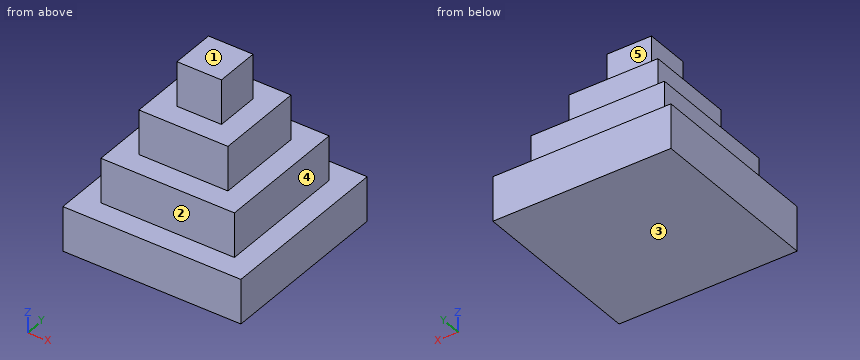
```python
from build123d import *

# Parameters (mm, degrees)
F1_W     = 25
F1_H     = 25
F1_W_2   = 18.75
F1_H_2   = 18.75
F2_DEPTH = 6.25
F1_W_3   = 12.5
F1_H_3   = 12.5
F3_DEPTH = 12.5
F1_W_4   = 6.25
F1_H_4   = 6.25
F4_DEPTH = 18.75
F5_DEPTH = 25


with BuildPart() as f2:
    # F1 (on Top) → F2 (new body)
    with BuildSketch(Plane.XY):
        with Locations((12.5, 12.5)):
            Rectangle(F1_W, F1_H)
        with Locations((12.5, 12.5)):
            Rectangle(F1_W_2, F1_H_2, mode=Mode.SUBTRACT)
    extrude(amount=F2_DEPTH)

    # F1 (on Top) → F3 (join)
    with BuildSketch(Plane.XY):
        with Locations((12.5, 12.5)):
            Rectangle(F1_W_2, F1_H_2)
        with Locations((12.5, 12.5)):
            Rectangle(F1_W_3, F1_H_3, mode=Mode.SUBTRACT)
    extrude(amount=F3_DEPTH)

    # F1 (on Top) → F4 (join)
    with BuildSketch(Plane.XY):
        with Locations((12.5, 12.5)):
            Rectangle(F1_W_3, F1_H_3)
        with Locations((12.5, 12.5)):
            Rectangle(F1_W_4, F1_H_4, mode=Mode.SUBTRACT)
    extrude(amount=F4_DEPTH)

    # F1 (on Top) → F5 (join)
    with BuildSketch(Plane.XY):
        with Locations((12.5, 12.5)):
            Rectangle(F1_W_4, F1_H_4)
    extrude(amount=F5_DEPTH)


solid = f2.part
```
Work out the finished part from the listing and answer in its coordinate system (mm). Face numbers are marked on the shaded views. A direction names the side the tool comes from. Round coordinates to 2 decimals unless told otherwise and drop trailing zeros. Order: outer loops, then holes, each group sorted by start corner. A loop starts at its lowest first (then second) coordinate and runs counter-clockwise, first axis right, second up.
Q1. Given pin 1 Ø3 at (x, y) = (4, 8.5) entering from +Z; pin 2 Ø1 at (x, z) = (14.5, 20) entering from +Y (3 decimals); pin 3 Ø5 at (y, z) = (12.5, 23.5) entering from +X (3 decimals), each flat-ended and moving along its own axis, determine where each tip first touches the part or whether it passes through.
Solution:
pin 1: stops at z = 12.5
pin 2: stops at y = 15.625
pin 3: stops at x = 15.625
Q2. Find the intervals of material crossed by line 1 along Z through (x, y) = (4, 22); line 2 along X through (y, z) = (10.5, 6.75) (3 decimals), in increasing order.
Solution:
line 1: z = 0 to 6.25
line 2: x = 3.125 to 21.875
Q3. A cutting plane is placed at A-A, the plane y = 18.25. Determine the outline of the cut face in (x, z) (3 decimals), then the cut area to 3 significant figures.
Solution:
outline: (0, 0) - (25, 0) - (25, 6.25) - (21.875, 6.25) - (21.875, 12.5) - (18.75, 12.5) - (18.75, 18.75) - (6.25, 18.75) - (6.25, 12.5) - (3.125, 12.5) - (3.125, 6.25) - (0, 6.25) - close
area: 352 mm2
Q4. A cutting plane is placed at B-B, the plane x = 12.5. Determine the outline of the cut face in (y, z) (3 decimals).
Solution:
outline: (0, 0) - (25, 0) - (25, 6.25) - (21.875, 6.25) - (21.875, 12.5) - (18.75, 12.5) - (18.75, 18.75) - (15.625, 18.75) - (15.625, 25) - (9.375, 25) - (9.375, 18.75) - (6.25, 18.75) - (6.25, 12.5) - (3.125, 12.5) - (3.125, 6.25) - (0, 6.25) - close
Q5. A tool of negligible diameter and unlimited length cuts with its end or side. For the marked faces 1, 2, 3, 4 and 5, from which of +Z, -Z, +X, -X, +Y, -Y can it reach the whole face along a straight path? Write none if from no direction.
Solution:
face 1: +Z, +X, -X, +Y, -Y
face 2: +Z, +X, -X, -Y
face 3: -Z, +X, -X, +Y, -Y
face 4: +Z, +X, +Y, -Y
face 5: +Z, +X, -X, +Y
Q6. A cutting plane is placed at D-D, the plane y = 21.5. Determine the outline of the cut face in (x, z) (3 decimals).
Solution:
outline: (0, 0) - (25, 0) - (25, 6.25) - (21.875, 6.25) - (21.875, 12.5) - (3.125, 12.5) - (3.125, 6.25) - (0, 6.25) - close
Q7. A cutting plane is placed at C-C, the plane z = 9.5. Determine the outline of the cut face in (x, y) (3 decimals), then the cut area to 3 significant figures.
Solution:
outline: (3.125, 3.125) - (21.875, 3.125) - (21.875, 21.875) - (3.125, 21.875) - close
area: 352 mm2
